Model file for the job. Use its own axes, mm. A direction names the side the tool comes from. Coordinates: 2 decimals unless noted, no trailing zeros. Write each loop counter-clockwise with the first axis right and the second up, starting at its lowest first coordinate (ties: lowest second). Pieces come first, ordered by that corner, then holes. Notation, with made-up numbers: M -9,52.25 L 40,52.25 A19 ccw 40,77.25 Z; hole C 29,-29 d6. An arc over 180 degrees is marked long. Use CSV: the item, a comma, the result in double quotes. Start each with the question number.
from build123d import *

# Parameters (mm, degrees)
BOSS_EXTRUDE1_DEPTH = 10
SKETCH3_W           = 20
SKETCH3_H           = 70
BOSS_EXTRUDE2_DEPTH = 20
SKETCH2_R           = 2.1
CUT_EXTRUDE1_DEPTH  = 79.74007874


with BuildPart() as part:
    # Sketch1 → Boss-Extrude1 (new, symmetric)
    with BuildSketch(Plane(origin=(0, 0, 0), x_dir=(1, 0, 0), z_dir=(0, 1, 0))):
        with BuildLine():
            Line((10, 0), (10, 10))
            ThreePointArc((10, 10), (12.928932188, 17.071067812), (20, 20))
            Line((20, 20), (30, 20))
            Line((30, 20), (30, 40))
            Line((30, 40), (20, 40))
            ThreePointArc((20, 40), (-1.213203436, 31.213203436), (-10, 10))
            Line((-10, 10), (-10, 0))
            Line((-10, 0), (10, 0))
        make_face()
    extrude(amount=BOSS_EXTRUDE1_DEPTH, both=True)

    # Sketch3 → Boss-Extrude2 (add)
    with BuildSketch(Plane(origin=(0, 10, 0), x_dir=(1, 0, 0), z_dir=(0, 1, 0))):
        with Locations((0, -35)):
            Rectangle(SKETCH3_W, SKETCH3_H)
    extrude(amount=-BOSS_EXTRUDE2_DEPTH)

    # Sketch2 → Cut-Extrude1 (cut, through all)
    with BuildSketch(Plane(origin=(0, 10, 0), x_dir=(1, 0, 0), z_dir=(0, 1, 0))):
        with Locations(Location((5.857864376, 24.142135624, 0), (0, 0, 270))):
            Circle(SKETCH2_R)
        with Locations(Location((0, -40, 0), (0, 0, 270))):
            Circle(SKETCH2_R)
        with Locations((70, 30)):
            Circle(SKETCH2_R)
        with Locations(Location((0, -60, 0), (0, 0, 270))):
            Circle(SKETCH2_R)
        with Locations(Location((0, -20, 0), (0, 0, 270))):
            Circle(SKETCH2_R)
        with Locations(Location((0, 0, 0), (0, 0, 270))):
            Circle(SKETCH2_R)
    extrude(amount=-CUT_EXTRUDE1_DEPTH, mode=Mode.SUBTRACT)

    # Mirror1: part across plane


with BuildPart() as part_1:
    add(part.part)
    add(part.part.mirror(Plane(origin=(10, -82.801098893, 70), x_dir=(1, 0, 0), z_dir=(0, 0, 1))))


solid = part_1.part
1) Two-plate mould, pull along X, no slides. Class faces 1 (the face through (25, 0, 160)), 2 (the face through (-0.979, 0.14, 171.445)), 3 (the face through (30, 0, 170)), 4 (the face through (0.09, 0.14, 102.1)): pulls with the +X half, pulls with the -X half, needs draft (parallel to the pull), parting line crosses it, or undercut.
2) Band-saw the part on B-B on x = 18. List the corners of the cut face in (y, z), then the cut area to 3 significant figures.
3) Band-saw the part on D-D on z = 4. List the corners of the cut face in (x, y), then the cut area to 3 significant figures.
4) Drop flat-ended pins along their axis: P1, Ø10, axis at x = 10, y = -1, coming from the +Z side; P2, Ø3, axis at y = -2.5, z = 137.5, coming from the +X side; P3, Ø2, axis at x = 13, y = 5, coming from the +Z side. Give the stop position or say it passes through.
5) Tool access for faces 5 (the face through (0.631, 0.14, 117.997)), 6 (the face through (12.85, 0.14, 156.99)): list every direction of +Z, -Z, +X, -X, +Y, -Y with a clear straight run to the whole face (end or side of a thin tool).
6) Wall check: L1, parallel to Z at x = 4.5, y = -6.25; L2, parallel to X at y = 5.5, z = 80; L3, parallel to Z at x = 22, y = 3.25. Give the ranges that are in metal, low to high. Write a range as [from, to].
7) Band-saw the part on C-C on y = -5.5. State how many separate pieces and enclosed holes the cut face has, then the cut area to 3 significant figures.
8) Band-saw the part on A-A on z = 140. List the corners of the cut face in (x, y).
Findings below:
1,face 1,"needs draft"
1,face 2,"pulls with the -X half"
1,face 3,"pulls with the +X half"
1,face 4,"undercut"
2,outline,"M -10,-39.93 L 10,-39.93 L 10,-19.8 L -10,-19.8 Z; M -10,159.8 L 10,159.8 L 10,179.93 L -10,179.93 Z"
2,area,"805 mm2"
3,outline,"M -10,-10 L 10,-10 L 10,10 L -10,10 Z"
3,area,"400 mm2"
4,P1,"stops at z = 179.58"
4,P2,"stops at x = 10"
4,P3,"stops at z = 179.39"
5,face 5,"+Y, -Y"
5,face 6,"+X, +Y, -Y"
6,L1,"z = [-35.69, -25.74], [-22.54, 162.54], [165.74, 175.69]"
6,L2,"x = [-10, -2.1], [2.1, 10]"
6,L3,"z = [-40, -20], [160, 180]"
7,separate pieces,"1"
7,enclosed holes,"10"
7,area,"4,720 mm2"
8,outline,"M -10,-10 L -2.1,-10 L -2.1,10 L -10,10 Z; M 2.1,-10 L 10,-10 L 10,10 L 2.1,10 Z"
